Work out the finished part from the listing and answer in its coordinate system (mm). Face numbers are marked on the shaded views. Coordinates: 2 decimals unless noted, no trailing zeros. Loops run counter-clockwise (first coordinate to the right, second up) from the corner with the lowest first, then second, coordinate; pieces in that order, holes last. Notation, with made-up numbers: (89.25, 48) -> (117.25, 48) arc R28 cw to (117.25, 81) -> close; hole circle Ø11 at (37.25, 4). An arc over 180 degrees is marked (long way). Use a Markdown table: item, result.
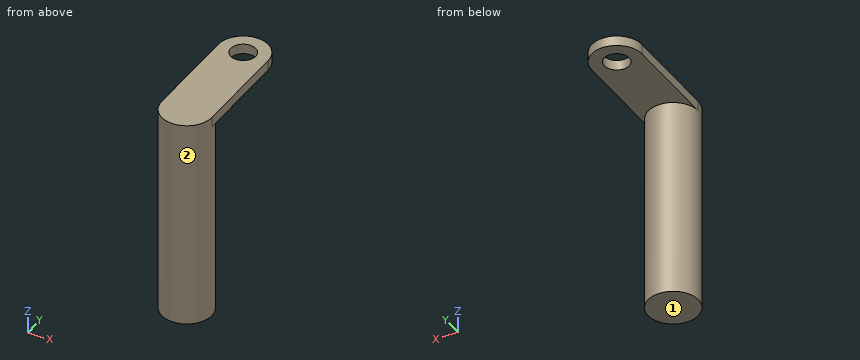
Autodesk Inventor part; units mm, degrees
ref_plane "YZ Plane" through (0, 0, 0) normal (1, 0, 0) x (0, 1, 0)
ref_plane "XZ Plane" through (0, 0, 0) normal (0, 1, 0) x (-1, 0, 0)
ref_plane "XY Plane" through (0, 0, 0) normal (0, 0, 1) x (1, 0, 0)
sketch "Sketch1" plane through (0, 0, 0) normal (0, 0, 1) x (1, 0, 0)
  circle A0 centre (0, 0) radius 6.35
  dimension "d0" = 12.7
extrude "Extrusion1" add sketch "Sketch1" along normal blind 50.8
sketch "Sketch2" plane through (0, 0, 50.8) normal (0, 0, 1) x (1, 0, 0)
  circle A0 centre (0, 0) radius 6.35
  line L0 (0, 0) -> (0, 25.4)
  circle A1 centre (0, 25.4) radius 6.35
  line L1 (-6.35, 25.4) -> (-6.35, 0)
  line L2 (6.35, 25.4) -> (6.35, 0)
  circle A2 centre (0, 25.4) radius 3.175
  dimension "d3" = 25.4
  dimension "d6" = 6.35
extrude "Extrusion2" add sketch "Sketch2" along normal blind 2.54
properties part number "main rack connection"
Q1. Determine the mould class of the marked faces 1 and 2 for opening direction Y: pulls with the +Y half, pulls with the -Y half, needs draft (parallel to the pull), parting line crosses it, or undercut.
Solved:
| item | result |
|---|---|
| face 1 | needs draft |
| face 2 | parting line crosses it |
Q2. Section A-A on x = 0 is taken. Determine the outline of the cut face in (y, z) (3 decimals).
Solved:
| item | result |
|---|---|
| outline | (-6.35, 0) -> (6.35, 0) -> (6.35, 50.8) -> (22.225, 50.8) -> (22.225, 53.34) -> (-6.35, 53.34) -> close; (28.575, 50.8) -> (31.75, 50.8) -> (31.75, 53.34) -> (28.575, 53.34) -> close |
Q3. Given pin 1 Ø5 at (x, y) = (-0.5, 1.5) entering from -Z; pin 2 Ø1 at (x, y) = (4.5, 23.5) entering from -Z; pin 3 Ø5 at (x, z) = (-2.5, 14) entering from +Y, each flat-ended and moving along its own axis, determine where each tip first touches the part or whether it passes through.
Solved:
| item | result |
|---|---|
| pin 1 | z = 0 |
| pin 2 | z = 50.8 |
| pin 3 | y = 6.35 |
Q4. Section D-D on x = -3.75 is taken. Determine the outline of the cut face in (y, z).
Solved:
| item | result |
|---|---|
| outline | (-5.12, 0) -> (5.12, 0) -> (5.12, 50.8) -> (30.52, 50.8) -> (30.52, 53.34) -> (-5.12, 53.34) -> close |
Q5. Consider line 1 (X direction, y = 25.4, z = 51.8) (3 decimals); line 2 (Y direction, x = 0, z = 51.4) (3 decimals); line 3 (Z direction, x = -1, y = 12). Determine where each line is inside the solid, lowest interval first. Write a range as [from, to].
Solved:
| item | result |
|---|---|
| line 1 | [-6.35, -3.175], [3.175, 6.35] |
| line 2 | [-6.35, 22.225], [28.575, 31.75] |
| line 3 | [50.8, 53.34] |
Q6. Section B-B on y = 3 is taken. Determine the outline of the cut face in (x, z).
Solved:
| item | result |
|---|---|
| outline | (-6.35, 50.8) -> (-5.6, 50.8) -> (-5.6, 0) -> (5.6, 0) -> (5.6, 50.8) -> (6.35, 50.8) -> (6.35, 53.34) -> (-6.35, 53.34) -> close |
Q7. Section C-C on z = 45.5 is taken. Determine the outline of the cut face in (x, y).
Solved:
| item | result |
|---|---|
| outline | circle Ø12.7 at (0, 0) |
